Model file for the job. Use its own axes, mm. A direction names the side the tool comes from. Round coordinates to 2 decimals unless told otherwise and drop trailing zeros. Loops run counter-clockwise (first coordinate to the right, second up) from the corner with the lowest first, then second, coordinate; pieces in that order, holes last. Notation, with made-up numbers: (87, 14.5) -> (144, 14.5) arc R28 cw to (144, 50.5) -> close; hole circle Ø5 at (-16, 42). An arc over 180 degrees is marked (long way). Use a Markdown table: item, result.
from build123d import *

# Parameters (mm, degrees)
SKETCH018_W     = 166
SKETCH018_H     = 166
PAD009_DEPTH    = 16
SKETCH019_W     = 160
SKETCH019_H     = 160
POCKET009_DEPTH = 13
SKETCH020_R     = 5
PAD010_DEPTH    = 12
SKETCH021_W     = 40
SKETCH021_H     = 10
POCKET010_DEPTH = 5
SKETCH022_W     = 46
SKETCH022_H     = 16
SKETCH022_W_2   = 40
SKETCH022_H_2   = 10
PAD011_DEPTH    = 5
CHAMFER001_SIZE = 2
FILLET004_R     = 0.6
SKETCH023_R     = 7
PAD012_DEPTH    = 5
SKETCH024_R     = 1.1
POCKET011_DEPTH = 166.001
SKETCH025_R     = 1.1
POCKET012_DEPTH = 167


with BuildPart() as part:
    # Sketch018 → Pad009 (new body)
    with BuildSketch(Plane.XY):
        with Locations((83, 83)):
            Rectangle(SKETCH018_W, SKETCH018_H)
    extrude(amount=PAD009_DEPTH)

    # Sketch019 (on Face6 of Pad009) → Pocket009 (cut)
    with BuildSketch(Plane.XY.offset(16)):
        with Locations((83, 83)):
            Rectangle(SKETCH019_W, SKETCH019_H)
    extrude(amount=-POCKET009_DEPTH, mode=Mode.SUBTRACT)

    # Sketch020 (on Face11 of Pocket009) → Pad010 (join)
    with BuildSketch(Plane.XY.offset(3)):
        with Locations((11, 155)):
            Circle(SKETCH020_R)
        with Locations((83, 155)):
            Circle(SKETCH020_R)
        with Locations((155, 155)):
            Circle(SKETCH020_R)
        with Locations((11, 83)):
            Circle(SKETCH020_R)
        with Locations((83, 83)):
            Circle(SKETCH020_R)
        with Locations((155, 83)):
            Circle(SKETCH020_R)
        with Locations((11, 11)):
            Circle(SKETCH020_R)
        with Locations((83, 11)):
            Circle(SKETCH020_R)
        with Locations((155, 11)):
            Circle(SKETCH020_R)
    extrude(amount=PAD010_DEPTH)

    # Sketch021 (on Face11 of Pad010) → Pocket010 (cut)
    with BuildSketch(Plane.XY.offset(3)):
        with Locations((83, 138)):
            Rectangle(SKETCH021_W, SKETCH021_H)
    extrude(amount=-POCKET010_DEPTH, mode=Mode.SUBTRACT)

    # Sketch022 (on Face15 of Pocket010) → Pad011 (join)
    with BuildSketch(Plane.XY.offset(3)):
        with Locations((83, 138)):
            Rectangle(SKETCH022_W, SKETCH022_H)
        with Locations((83, 138)):
            Rectangle(SKETCH022_W_2, SKETCH022_H_2, mode=Mode.SUBTRACT)
    extrude(amount=PAD011_DEPTH)

    # Chamfer001
    chamfer001_edges = [part.edges().sort_by_distance(p)[0] for p in [
        (83, 130, 3),
        (60, 138, 3),
        (106, 138, 3),
        (83, 146, 3),
    ]]
    chamfer(chamfer001_edges, length=CHAMFER001_SIZE)

    # Fillet004
    fillet004_edges = [part.edges().sort_by_distance(p)[0] for p in [
        (83, 146, 8),
        (106, 138, 8),
        (83, 130, 8),
        (60, 138, 8),
        (83, 143, 8),
        (103, 138, 8),
        (83, 133, 8),
        (63, 138, 8),
    ]]
    fillet(fillet004_edges, radius=FILLET004_R)

    # Sketch023 (on Face11 of Fillet004) → Pad012 (join)
    with BuildSketch(Plane.XY.offset(3)):
        with Locations((11, 155)):
            Circle(SKETCH023_R)
        with Locations((83, 155)):
            Circle(SKETCH023_R)
        with Locations((155, 155)):
            Circle(SKETCH023_R)
        with Locations((11, 83)):
            Circle(SKETCH023_R)
        with Locations((83, 83)):
            Circle(SKETCH023_R)
        with Locations((155, 83)):
            Circle(SKETCH023_R)
        with Locations((11, 11)):
            Circle(SKETCH023_R)
        with Locations((83, 11)):
            Circle(SKETCH023_R)
        with Locations((155, 11)):
            Circle(SKETCH023_R)
    extrude(amount=PAD012_DEPTH)

    # Sketch024 (on Face50 of Pad012) → Pocket011 (cut, through all)
    with BuildSketch(Plane.XZ):
        with Locations((39.899256, 3)):
            Circle(SKETCH024_R)
        with Locations((119.697768, 6)):
            Circle(SKETCH024_R)
    extrude(amount=-POCKET011_DEPTH, mode=Mode.SUBTRACT)

    # Sketch025 (on Face48 of Pocket011) → Pocket012 (cut)
    with BuildSketch(Plane.YZ.offset(166)):
        with Locations((41.5, 3)):
            Circle(SKETCH025_R)
        with Locations((124.5, 3)):
            Circle(SKETCH025_R)
    extrude(amount=-POCKET012_DEPTH, mode=Mode.SUBTRACT)


solid = part.part
Q1. Drill centre lines: L1, parallel to Y at x = 112, z = 12; L2, parallel to X at y = 10.5, z = 14.25; L3, parallel to Y at x = 150.5, z = 3.5. Where is each one in solid material? Low to high. Write a range as from..to.
Results list:
| item | result |
|---|---|
| L1 | y = 0..3, 163..166 |
| L2 | x = 0..3, 6.03..15.97, 78.03..87.97, 150.03..159.97, 163..166 |
| L3 | y = 0..3, 5.64..16.36, 77.64..88.36, 149.64..160.36, 163..166 |
Q2. Band-saw the part on B-B, the plane y = 23. Give the cut face in (x, z).
Results list:
| item | result |
|---|---|
| outline | (0, 0) -> (166, 0) -> (166, 16) -> (163, 16) -> (163, 3) -> (41, 3) arc R1.1 cw to (38.8, 3) -> (3, 3) -> (3, 16) -> (0, 16) -> close |
Q3. Flat gauge pins, fed straight in: pin 1 (12 mm diameter, centred on x = 55.5, y = 61.5, fed in from +Z); pin 2 (11 mm diameter, centred on x = 13, y = 85.5, fed in from +Z); pin 3 (2 mm diameter, centred on y = 124.5, z = 3, fed in from +X); pin 4 (12 mm diameter, centred on x = 78.5, y = 140, fed in from +Z). Where does each tip first touch, or does it go through?
Results list:
| item | result |
|---|---|
| pin 1 | stops at z = 3 |
| pin 2 | stops at z = 15 |
| pin 3 | passes through |
| pin 4 | stops at z = 8 |
Q4. Tool access for faces 1 (the face through (155, 11, 15)), 2 (the face through (83, 143, 4)): list every direction of +Z, -Z, +X, -X, +Y, -Y with a clear straight run to the whole face (end or side of a thin tool).
Results list:
| item | result |
|---|---|
| face 1 | +Z |
| face 2 | +Z, -Z |
Q5. Pull direction X, two halves, no side cores. Call faces 3 (the face through (0, 82, 8)), 4 (the face through (2.7, 120.3, 16)), 5 (the face through (150, 11, 11)): released by +X, released by -X, zero draft, split by the parting line, or undercut.
Results list:
| item | result |
|---|---|
| face 3 | released by -X |
| face 4 | zero draft |
| face 5 | undercut |
Q6. Band-saw the part on A-A, the plane x = 54.5. Give the cut face in (y, z).
Results list:
| item | result |
|---|---|
| outline | (0, 0) -> (166, 0) -> (166, 16) -> (163, 16) -> (163, 3) -> (125.6, 3) arc R1.1 cw to (123.4, 3) -> (42.6, 3) arc R1.1 cw to (40.4, 3) -> (3, 3) -> (3, 16) -> (0, 16) -> close |
